from build123d import *

# Parameters (mm, degrees)
F0_R     = 39.7326130333
F1_DEPTH = 76.2
F1_TAPER = -3
F2_T     = -2.54
F3_DEPTH = 25.4
F4_T     = -2.54
F5_R     = 18.2833455915
F6_DEPTH = 25.4
F7_R     = 7.4141197659
F8_DEPTH = 88.9


with BuildPart() as f1:
    # F0 (on Top) → F1 (new body)
    with BuildSketch(Plane.XY):
        Circle(F0_R)
    extrude(amount=F1_DEPTH, taper=F1_TAPER)

    # F2
    f2_openings = [f1.faces().sort_by_distance(p)[0] for p in [
        (0, 0, 76.2),
    ]]
    offset(amount=F2_T, openings=f2_openings, kind=Kind.INTERSECTION)

    # F3 (add): a face of the model
    f3_faces = [f1.faces().sort_by_distance(p)[0] for p in [
        (0, 0, 2.54),
    ]]
    extrude(f3_faces, amount=F3_DEPTH)

    # F4
    f4_openings = [f1.faces().sort_by_distance(p)[0] for p in [
        (0, 0, 27.94),
    ]]
    offset(amount=F4_T, openings=f4_openings, kind=Kind.INTERSECTION)

    # F5 (on Top) → F6 (join)
    with BuildSketch(Plane.XY):
        Circle(F5_R)
    extrude(amount=F6_DEPTH)

    # F7 (on Top) → F8 (join)
    with BuildSketch(Plane.XY):
        Circle(F7_R)
    extrude(amount=F8_DEPTH)


solid = f1.part
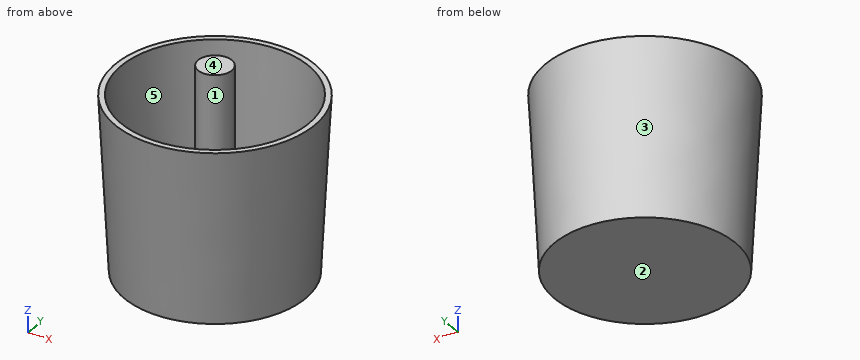
CAD build for the part. Positions are in the model's coordinates, mm. Face numbers are marked on the shaded views. A direction names the side the tool comes from. Round coordinates to 2 decimals unless told otherwise and drop trailing zeros. Write each loop counter-clockwise with the first axis right and the second up, starting at its lowest first coordinate (ties: lowest second). Pieces come first, ordered by that corner, then holes.
(1) Slice it at B-B, the plane z = 31. Write the cut outline in (x, y), and give its area (3 significant figures).
(2) Slice it at A-A, the plane x = 0. Write the cut outline in (y, z), and give its area (3 significant figures).
(3) Mould opens along X. For the marked faces 3, 4 and 5 say: pulls with the +X half, pulls with the -X half, needs draft (parallel to the pull), parting line crosses it, or undercut.
(4) Slice it at C-C, the plane z = 80. Write the cut outline in (x, y).
(5) 3-axis set-ups, long thin cutter, end or side, ignore diameter. For the marked faces 1 and 2: which of +Z, -Z, +X, -X, +Y, -Y reach the whole face in a straight line?
(6) Probe line 1 along X through (y, z) = (30, 4.5); line 2 along Y through (x, z) = (-28, 23); line 3 along Y through (x, z) = (0, 9). List the from-to ranges inside material, lowest first.
(7) Drop flat-ended pins along their axis: P1, Ø3, axis at x = 25.5, z = 73.5, coming from the -Y side; P2, Ø5, axis at y = 34, z = 70.5, coming from the -X side; P3, Ø8, axis at x = 10.5, y = 7.5, coming from the -Z side; P4, Ø10, axis at x = 30, y = -10, coming from the +Z side. Give the stop position or say it passes through.
From the geometry:
1. outline: circle Ø82.71 at (0, 0); circle Ø14.83 at (0, 0); hole circle Ø77.63 at (0, 0)
1. area: 813 mm2
2. outline: (-43.73, 76.2) - (-39.73, 0) - (39.73, 0) - (43.73, 76.2) - (41.18, 76.2) - (37.32, 2.54) - (37.32, 27.94) - (34.78, 27.94) - (34.78, 2.54) - (18.28, 2.54) - (18.28, 25.4) - (7.41, 25.4) - (7.41, 88.9) - (-7.41, 88.9) - (-7.41, 25.4) - (-18.28, 25.4) - (-18.28, 2.54) - (-34.78, 2.54) - (-34.78, 27.94) - (-37.32, 27.94) - (-37.32, 2.54) - (-41.18, 76.2) - close
2. area: 2,480 mm2
3. face 3: parting line crosses it
3. face 4: needs draft
3. face 5: undercut
4. outline: circle Ø14.83 at (0, 0)
5. face 1: +Z
5. face 2: -Z, +X, -X, +Y, -Y
6. line 1: x = -26.41 to -22.37, -22.2 to -17.6, 17.6 to 22.2, 22.37 to 26.41
6. line 2: y = -29.87 to -26.27, -24.68 to -20.64, 20.64 to 24.68, 26.27 to 29.87
6. line 3: y = -40.2 to -37.66, -37.32 to -34.78, -18.28 to 18.28, 34.78 to 37.32, 37.66 to 40.2
7. P1: stops at y = -36.39
7. P2: stops at x = -29.9
7. P3: stops at z = 0
7. P4: stops at z = 27.94
